Can you work these out from the model? Positions are in its coordinate system, mm. A direction names the side the tool comes from. Coordinates: 2 decimals unless noted, no trailing zeros. Loops run counter-clockwise (first coordinate to the right, second up) from the corner with the lowest first, then second, coordinate; pieces in that order, holes last. Notation, with made-up numbers: (12, -26.5) -> (62, -26.5) arc R21 cw to (62, 0.5) -> close; hole circle Ø9 at (35, 20). An arc over 180 degrees is marked (long way). Use one line per item in the form item = value. Start each with the question number.
(1) Imagine slicing it at A-A (y = 12). List the corners of the cut face in (x, z) for me (3 decimals).
(2) Imagine slicing it at D-D (x = 7.5). List the corners of the cut face in (y, z) for me.
(3) Thinking about a two-plate mould opening in Z: for faces 1 (the flat face through (0, 8, -23)), 2 (the flat face through (0, 9, -6)), 3 (the cylindrical face through (27.064, 7.395, -5.464)), 4 (the cylindrical face through (-29.936, 9.624, -18.464)), which applies, released by +Z, released by -Z, zero draft, split by the parting line, or undercut?
(4) I'm going to push flat-ended pins straight in: pin 1 (8 mm diameter, centred on x = 0.5, z = -7.5, fed in from +Y); pin 2 (1.5 mm diameter, centred on x = 26, z = -9, fed in from -Y); pin 3 (10 mm diameter, centred on x = 28.5, z = 10, fed in from +Y); pin 4 (10 mm diameter, centred on x = -28.5, z = -15, fed in from +Y). Where does each tip first touch, or does it pass through?
(5) On a 3-axis mill with a long thin cutter (end or side, diameter ignored), from which of +Z, -Z, +X, -X, +Y, -Y can I reach the whole of each face in a straight line? I mean faces 5 (the flat face through (34, 8, -5)), 6 (the flat face through (22, 12, -13)). Say none if no direction works.
(6) Imagine slicing it at C-C (z = -15). List the corners of the cut face in (x, y) for me.
(7) I need wall thicknesses on line 1 (Z direction, x = 28.5, y = 8.25); line 2 (X direction, y = 3.75, z = 10); line 3 (X direction, y = 14.25, z = -15). Which ranges of each line are inside material? Lowest first, please. Write a range as [from, to].
(8) Imagine slicing it at B-B (x = -28.5). List the corners of the cut face in (y, z) for me.
```python
from build123d import *

# Parameters (mm, degrees)
SKETCH1_W           = 68
SKETCH1_H           = 46
BOSS_EXTRUDE1_DEPTH = 67
SKETCH3_W           = 44
SKETCH3_H           = 46
CUT_EXTRUDE2_DEPTH  = 58
CUT_EXTRUDE1_REACH  = 100.194
CUT_EXTRUDE3_REACH  = 48.109
SKETCH4_R           = 3.75


with BuildPart() as part:
    # Sketch1 → Boss-Extrude1 (new body)
    with BuildSketch(Plane(origin=(0, 0, 0), x_dir=(1, 0, 0), z_dir=(0, 1, 0))):
        Rectangle(SKETCH1_W, SKETCH1_H)
    extrude(amount=BOSS_EXTRUDE1_DEPTH)

    # Sketch3 → Cut-Extrude2 (cut)
    with BuildSketch(Plane(origin=(0, 67, 0), x_dir=(1, 0, 0), z_dir=(0, 1, 0))):
        Rectangle(SKETCH3_W, SKETCH3_H)
    extrude(amount=-CUT_EXTRUDE2_DEPTH, mode=Mode.SUBTRACT)

    # Cut-Extrude1: up to this face of the body (flat: up to its plane)
    cut_extrude1_end = Plane(part.part.faces().sort_by_distance((-34, 33.5, 0))[0])
    # Sketch2 → Cut-Extrude1 (cut, up to the picked face)
    with BuildSketch(Plane(origin=(34, 0, 0), x_dir=(0, 0, -1), z_dir=(1, 0, 0)), mode=Mode.PRIVATE) as cut_extrude1_sk1:
        Polygon((-23, 5), (23, 21), (23, 67), (-23, 67), align=None)
    cut_extrude1_tool1 = split(extrude(cut_extrude1_sk1.sketch, amount=-CUT_EXTRUDE1_REACH, mode=Mode.PRIVATE), bisect_by=cut_extrude1_end, keep=Keep.BOTH, mode=Mode.PRIVATE)
    add(cut_extrude1_tool1.solids().sort_by(Axis((34, 39.802469, 1.135802), (-1, 0, 0)))[0], mode=Mode.SUBTRACT)

    # Cut-Extrude3: up to this plane
    cut_extrude3_end = Plane(origin=(-111.201036262, 5, 23), z_dir=(0, -0.9444967967061592, -0.32852062494127277))
    # Sketch4 → Cut-Extrude3 (cut, up to the surface)
    with BuildSketch(Plane(origin=(0, 0, 0), x_dir=(-1, 0, 0), z_dir=(0, -1, 0)), mode=Mode.PRIVATE) as cut_extrude3_sk1:
        with Locations(Location((-28.5, 15, 0), (0, 0, 90))):
            Circle(SKETCH4_R)
    cut_extrude3_tool1 = split(extrude(cut_extrude3_sk1.sketch, amount=-CUT_EXTRUDE3_REACH, mode=Mode.PRIVATE), bisect_by=cut_extrude3_end, keep=Keep.BOTH, mode=Mode.PRIVATE)
    add(cut_extrude3_tool1.solids().sort_by_distance((28.5, 0, -15))[0], mode=Mode.SUBTRACT)
    # Sketch4 → Cut-Extrude3 (cut, up to the surface)
    with BuildSketch(Plane(origin=(0, 0, 0), x_dir=(-1, 0, 0), z_dir=(0, -1, 0)), mode=Mode.PRIVATE) as cut_extrude3_sk2:
        with Locations(Location((-28.5, 2, 0), (0, 0, 90))):
            Circle(SKETCH4_R)
    cut_extrude3_tool2 = split(extrude(cut_extrude3_sk2.sketch, amount=-CUT_EXTRUDE3_REACH, mode=Mode.PRIVATE), bisect_by=cut_extrude3_end, keep=Keep.BOTH, mode=Mode.PRIVATE)
    add(cut_extrude3_tool2.solids().sort_by_distance((28.5, 0, -2))[0], mode=Mode.SUBTRACT)
    # Sketch4 → Cut-Extrude3 (cut, up to the surface)
    with BuildSketch(Plane(origin=(0, 0, 0), x_dir=(-1, 0, 0), z_dir=(0, -1, 0)), mode=Mode.PRIVATE) as cut_extrude3_sk3:
        with Locations(Location((-28.5, -10, 0), (0, 0, 90))):
            Circle(SKETCH4_R)
    cut_extrude3_tool3 = split(extrude(cut_extrude3_sk3.sketch, amount=-CUT_EXTRUDE3_REACH, mode=Mode.PRIVATE), bisect_by=cut_extrude3_end, keep=Keep.BOTH, mode=Mode.PRIVATE)
    add(cut_extrude3_tool3.solids().sort_by_distance((28.5, 0, 10))[0], mode=Mode.SUBTRACT)
    # Sketch4 → Cut-Extrude3 (cut, up to the surface)
    with BuildSketch(Plane(origin=(0, 0, 0), x_dir=(-1, 0, 0), z_dir=(0, -1, 0)), mode=Mode.PRIVATE) as cut_extrude3_sk4:
        with Locations(Location((28.5, 15, 0), (0, 0, 90))):
            Circle(SKETCH4_R)
    cut_extrude3_tool4 = split(extrude(cut_extrude3_sk4.sketch, amount=-CUT_EXTRUDE3_REACH, mode=Mode.PRIVATE), bisect_by=cut_extrude3_end, keep=Keep.BOTH, mode=Mode.PRIVATE)
    add(cut_extrude3_tool4.solids().sort_by_distance((-28.5, 0, -15))[0], mode=Mode.SUBTRACT)
    # Sketch4 → Cut-Extrude3 (cut, up to the surface)
    with BuildSketch(Plane(origin=(0, 0, 0), x_dir=(-1, 0, 0), z_dir=(0, -1, 0)), mode=Mode.PRIVATE) as cut_extrude3_sk5:
        with Locations(Location((28.5, 2, 0), (0, 0, 90))):
            Circle(SKETCH4_R)
    cut_extrude3_tool5 = split(extrude(cut_extrude3_sk5.sketch, amount=-CUT_EXTRUDE3_REACH, mode=Mode.PRIVATE), bisect_by=cut_extrude3_end, keep=Keep.BOTH, mode=Mode.PRIVATE)
    add(cut_extrude3_tool5.solids().sort_by_distance((-28.5, 0, -2))[0], mode=Mode.SUBTRACT)
    # Sketch4 → Cut-Extrude3 (cut, up to the surface)
    with BuildSketch(Plane(origin=(0, 0, 0), x_dir=(-1, 0, 0), z_dir=(0, -1, 0)), mode=Mode.PRIVATE) as cut_extrude3_sk6:
        with Locations(Location((28.5, -10, 0), (0, 0, 90))):
            Circle(SKETCH4_R)
    cut_extrude3_tool6 = split(extrude(cut_extrude3_sk6.sketch, amount=-CUT_EXTRUDE3_REACH, mode=Mode.PRIVATE), bisect_by=cut_extrude3_end, keep=Keep.BOTH, mode=Mode.PRIVATE)
    add(cut_extrude3_tool6.solids().sort_by_distance((-28.5, 0, 10))[0], mode=Mode.SUBTRACT)


solid = part.part
```
Worked out:
q1.outline = (-34, -23) -> (-22, -23) -> (-22, 2.875) -> (-34, 2.875) -> close; (22, -23) -> (34, -23) -> (34, 2.875) -> (22, 2.875) -> close; hole circle Ø7.5 at (-28.5, -15); hole circle Ø7.5 at (-28.5, -2); hole circle Ø7.5 at (28.5, -15); hole circle Ø7.5 at (28.5, -2)
q2.outline = (0, -23) -> (9, -23) -> (9, 11.5) -> (5, 23) -> (0, 23) -> close
q3.face_1 = released by -Z
q3.face_2 = zero draft
q3.face_3 = undercut
q3.face_4 = undercut
q4.pin_1 = 9
q4.pin_2 = 0
q4.pin_3 = 11.26
q4.pin_4 = 19.96
q5.face_5 = +Z, -Z, +X, +Y, -Y
q5.face_6 = +Z, -Z, +Y
q6.outline = (-34, 0) -> (-32.25, 0) -> (-32.25, 18.22) -> (-34, 18.22) -> close; (-24.75, 0) -> (24.75, 0) -> (24.75, 18.22) -> (22, 18.22) -> (22, 9) -> (-22, 9) -> (-22, 18.22) -> (-24.75, 18.22) -> close; (32.25, 0) -> (34, 0) -> (34, 18.22) -> (32.25, 18.22) -> close
q7.line_1 = [-23, -18.75], [-11.25, -5.75], [1.75, 6.25]
q7.line_2 = [-34, -32.25], [-24.75, 24.75], [32.25, 34]
q7.line_3 = [-34, -32.25], [-24.75, -22], [22, 24.75], [32.25, 34]
q8.outline = (0, -23) -> (21, -23) -> (19.52, -18.75) -> (0, -18.75) -> close; (0, -11.25) -> (16.91, -11.25) -> (15, -5.75) -> (0, -5.75) -> close; (0, 1.75) -> (12.39, 1.75) -> (10.83, 6.25) -> (0, 6.25) -> close; (0, 13.75) -> (8.22, 13.75) -> (5, 23) -> (0, 23) -> close
